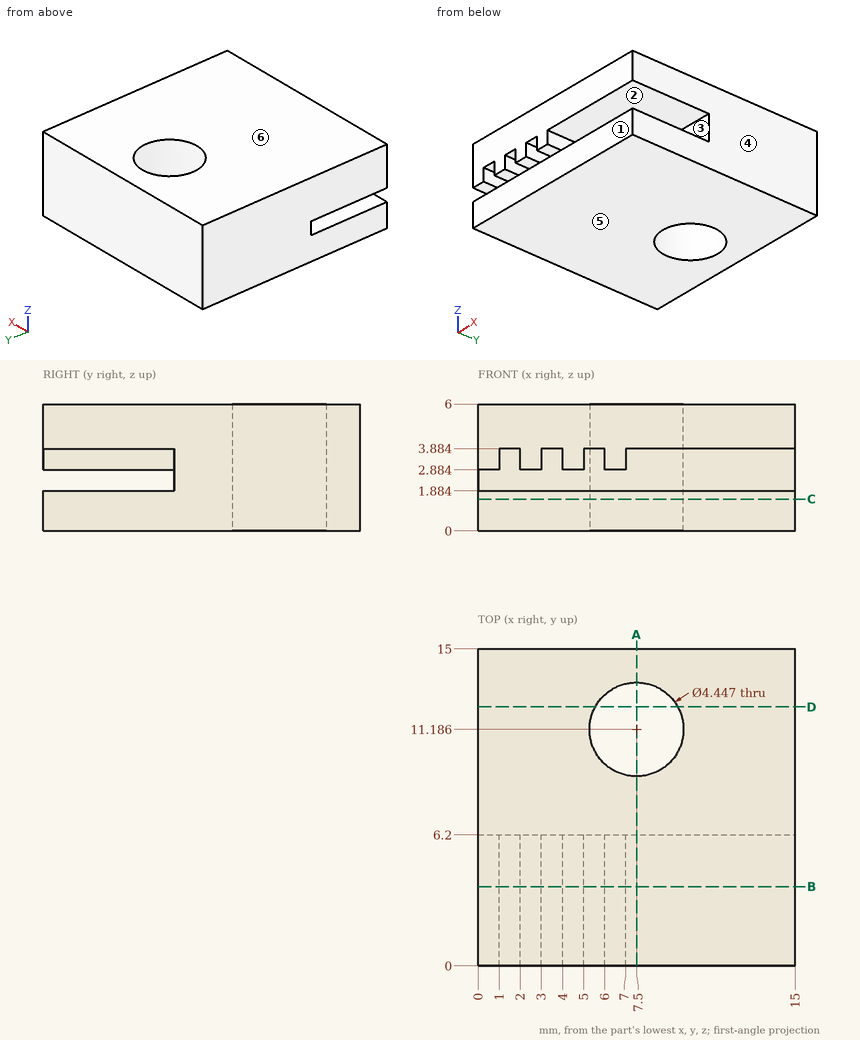
Here's the drawing with two shaded views (mm, measured from the low corner). I have some questions. A direction names the side the tool comes from. Give positions to 0.01 mm unless a question says otherwise; leave off trailing zeros. Write each loop counter-clockwise with the first axis right and the second up, starting at its lowest first coordinate (ties: lowest second). Pieces come first, ordered by that corner, then holes. Notation, with made-up numbers: (80, -8.75) - (104, -8.75) arc R9 cw to (104, 2.25) - close; hole circle Ø1 at (73, 76.25). An arc over 180 degrees is marked (long way). One line per item, written item: value. Start each with the question number.
Item 1: Imagine slicing it at D-D, the plane y = 12.25. List the corners of the cut face in (x, z) for me.
Item 2: If we mould it in two halves opening along Z, with no side actions, what happens to the marked faces 3, 4, 5 and 6? For each: +Z half, -Z half, draft (parallel to the pull), parting line (faces both ways), or undercut.
Item 3: Imagine slicing it at C-C, the plane z = 1.5. List the corners of the cut face in (x, y) for me (1 decimal).
Item 4: Imagine slicing it at A-A, the plane x = 7.5. List the corners of the cut face in (y, z) for me.
Item 5: Which directions (+Z, -Z, +X, -X, +Y, -Y) give clear straight access to the entire face, cutting with the end or side of a thin tool? Please do the marked faces 1 and 2.
Item 6: Please list where these lines run through material, in increasing order: line 1 (Z direction, x = 3.75, y = 1); line 2 (Y direction, x = 7.5, z = 2.8); line 3 (Y direction, x = 7.5, z = 4.1). Write a range as from..to.
Item 7: Imagine slicing it at B-B, the plane y = 3.75. List the corners of the cut face in (x, z) for me.
Geometry says:
1. outline: (0, 0) - (5.55, 0) - (5.55, 6) - (0, 6) - close; (9.45, 0) - (15, 0) - (15, 6) - (9.45, 6) - close
2. face 3: undercut
2. face 4: draft
2. face 5: -Z half
2. face 6: +Z half
3. outline: (0, 0) - (15, 0) - (15, 15) - (0, 15) - close; hole circle Ø4.4 at (7.5, 11.2)
4. outline: (0, 0) - (8.96, 0) - (8.96, 6) - (0, 6) - (0, 3.88) - (6.2, 3.88) - (6.2, 1.88) - (0, 1.88) - close; (13.41, 0) - (15, 0) - (15, 6) - (13.41, 6) - close
5. face 1: +Z, -Z, +X, -X, -Y
5. face 2: +X, -Y
6. line 1: 0..1.88, 3.88..6
6. line 2: 6.2..8.96, 13.41..15
6. line 3: 0..8.96, 13.41..15
7. outline: (0, 0) - (15, 0) - (15, 1.88) - (0, 1.88) - close; (0, 2.88) - (1, 2.88) - (1, 3.88) - (2, 3.88) - (2, 2.88) - (3, 2.88) - (3, 3.88) - (4, 3.88) - (4, 2.88) - (5, 2.88) - (5, 3.88) - (6, 3.88) - (6, 2.88) - (7, 2.88) - (7, 3.88) - (15, 3.88) - (15, 6) - (0, 6) - close
